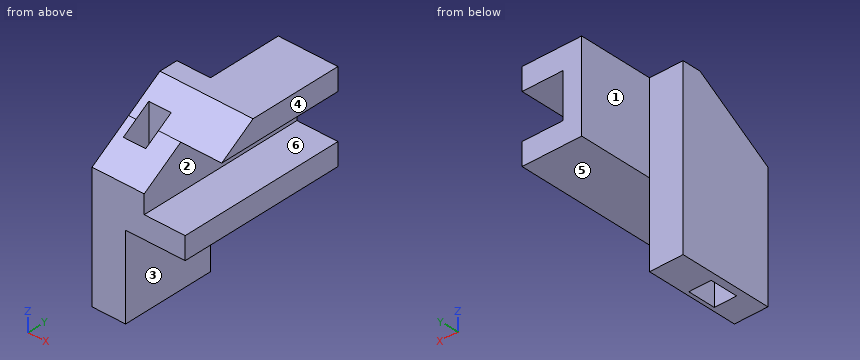
Solid Edge part; units mm, degrees
sketch "Sketch1" plane through (0, 0, 0) normal (0, 0, 1) x (1, 0, 0)
  line L0 (-175.9492, -30.1726) -> (-125.9492, -30.1726)
  line L1 (-175.9492, 59.8274) -> (-175.9492, -30.1726)
  line L2 (-125.9492, 59.8274) -> (-175.9492, 59.8274)
  line L3 (-125.9492, -30.1726) -> (-125.9492, 59.8274)
extrude "Protrusion1" add sketch "Sketch1" along normal blind 93
sketch "Sketch2" plane through (-150.9492, -30.1726, 46.5) normal (0, -1, 0) x (1, 0, 0)
  line L0 (25, -46.5) -> (-7, -46.5)
  line L1 (-7, -46.5) -> (-7, -1.5)
  line L2 (-7, -1.5) -> (25, -1.5)
  line L3 (25, -1.5) -> (25, -46.5)
extrude "ExtrudedCutout_1" cut sketch "Sketch2" along normal mid plane 366
sketch "Sketch3" plane through (-157.9492, 14.8274, 22.5) normal (1, 0, 0) x (0, 1, 0)
  line L0 (45, -22.5) -> (5, -22.5)
  line L1 (5, -22.5) -> (5, 22.5)
  line L2 (5, 22.5) -> (45, 22.5)
  line L3 (45, 22.5) -> (45, -22.5)
extrude "ExtrudedCutout_2" cut sketch "Sketch3" along normal mid plane 188
sketch "Sketch4" plane through (-150.9492, -30.1726, 46.5) normal (0, -1, 0) x (1, 0, 0)
  line L0 (25, 10.5) -> (3, 10.5)
  line L1 (3, 10.5) -> (3, 34.5)
  line L2 (3, 34.5) -> (25, 34.5)
  line L3 (25, 34.5) -> (25, 10.5)
extrude "ExtrudedCutout_3" cut sketch "Sketch4" along normal mid plane 238
sketch "Sketch5" plane through (-147.9492, 14.8274, 69) normal (1, 0, 0) x (0, 1, 0)
  line L0 (-45, 12) -> (-23.4615, 12)
  line L1 (-45, -2) -> (-23.4615, 12)
  line L2 (-45, -2) -> (-45, 12)
extrude "ExtrudedCutout_4" cut sketch "Sketch5" along normal mid plane 92
sketch "Sketch6" plane through (-125.9492, 14.8274, 87) normal (1, 0, 0) x (0, 1, 0)
  line L0 (-5, 6) -> (-23.4643, -6)
  line L1 (-23.4643, -6) -> (-45, -6)
  line L2 (-45, -6) -> (-45, 6)
  line L3 (-45, 6) -> (-5, 6)
extrude "ExtrudedCutout_5" cut sketch "Sketch6" along normal mid plane 122
sketch "Sketch7" plane through (-175.9492, 14.8274, 46.5) normal (-1, 0, 0) x (0, -1, 0)
  line L0 (-5, -1.5) -> (-5, 46.5)
  line L1 (-5, 46.5) -> (-45, 46.5)
  line L2 (-45, 46.5) -> (-45, -1.5)
  line L3 (-45, -1.5) -> (-5, -1.5)
extrude "Cutout_6" cut sketch "Sketch7" against normal blind 18
sketch "Sketch8" plane through (-150.9492, 34.8274, 93) normal (0, 0, 1) x (1, 0, 0)
  line L0 (-9, -50.9615) -> (-21, -50.9615)
  line L1 (-21, -50.9615) -> (-21, -43.4615)
  line L2 (-21, -43.4615) -> (-21, -35.9615)
  line L3 (-21, -35.9615) -> (-9, -35.9615)
  line L4 (-9, -35.9615) -> (-9, -50.9615)
extrude "Cutout_7" cut sketch "Sketch8" against normal blind 115
For this review, take the finished solid that the model builds, in its own axes (mm). Face numbers are marked on the shaded views. A direction names the side the tool comes from. Round coordinates to 2 decimals unless told otherwise and drop trailing zeros. Loops run counter-clockwise (first coordinate to the right, second up) from the corner with the lowest first, then second, coordinate; pieces in that order, holes last.
(1) Mouldability with a two-part tool opening along Z and no side actions: class the marked faces 4, 5 and 6 as released by +Z, released by -Z, zero draft, split by the parting line, or undercut.
Returned:
face 4: zero draft
face 5: released by -Z
face 6: undercut
(2) We need section C-C (z = 54). Give the boundary of the cut face in (x, y), plus the area to 3 significant figures.
Returned:
outline: (-175.95, -30.17) - (-125.95, -30.17) - (-125.95, 59.83) - (-157.95, 59.83) - (-157.95, 19.83) - (-175.95, 19.83) - close; hole (-171.95, -16.13) - (-159.95, -16.13) - (-159.95, -1.13) - (-171.95, -1.13) - close
area: 3,600 mm2
(3) We need section D-D (y = -4). Give the boundary of the cut face in (x, z), plus the area to 3 significant figures.
Returned:
outline: (-175.95, 0) - (-171.95, 0) - (-171.95, 84.01) - (-175.95, 84.01) - close; (-159.95, 0) - (-157.95, 0) - (-157.95, 45) - (-125.95, 45) - (-125.95, 57) - (-147.95, 57) - (-147.95, 81) - (-125.95, 81) - (-125.95, 84.01) - (-159.95, 84.01) - close
area: 1,220 mm2
(4) Clearance check with flat-ended pins moving along their axes: P1, Ø5, axis at y = 35.5, z = 70.5, coming from the +X side; P2, Ø12, axis at y = 47.5, z = 76, coming from the -X side; P3, Ø6, axis at x = -144, y = -6, coming from the +Z side; P4, Ø24, axis at x = -137.5, y = 0, coming from the +Z side. State where each tip first meets the part, or that it passes through.
Returned:
P1: stops at x = -147.95
P2: stops at x = -157.95
P3: stops at z = 84.66
P4: stops at z = 93
(5) We need section B-B (y = 43.5). Give the boundary of the cut face in (x, z).
Returned:
outline: (-157.95, 45) - (-125.95, 45) - (-125.95, 57) - (-147.95, 57) - (-147.95, 81) - (-125.95, 81) - (-125.95, 93) - (-157.95, 93) - close
(6) We need section A-A (x = -165.5). Give the boundary of the cut face in (y, z) (3 decimals).
Returned:
outline: (-30.173, 0) - (-16.134, 0) - (-16.134, 76.125) - (-30.173, 67) - close; (-1.134, 0) - (19.827, 0) - (19.827, 93) - (9.827, 93) - (-1.134, 85.876) - close
(7) Wall thickness on line 1 along Y through (x, z) = (-164, 42.5); line 2 along X through (y, z) = (-9, 62); line 3 along X through (y, z) = (-13, 49.5): over which ranges is each line inside the solid? List them lowest first.
Returned:
line 1: y = -30.17 to -16.13, -1.13 to 19.83
line 2: x = -175.95 to -171.95, -159.95 to -147.95
line 3: x = -175.95 to -171.95, -159.95 to -125.95
(8) Tool access review of the marked faces 1, 2 and 3: name each direction out of +Z, -Z, +X, -X, +Y, -Y from which nothing blocks a thin tool from reaching the whole face with its end or side.
Returned:
face 1: +Z, -Z, -X, +Y
face 2: +X, +Y, -Y
face 3: -Z, +X, +Y, -Y
